Drawing for the job (mm, zero at the part's lowest x, y, z). A direction names the side the tool comes from. Round coordinates to 2 decimals unless told otherwise and drop trailing zeros. Loops run counter-clockwise (first coordinate to the right, second up) from the corner with the lowest first, then second, coordinate; pieces in that order, holes last. Notation, with made-up numbers: (61.5, 32) - (75.5, 32) arc R21 cw to (75.5, 61) - close; hole circle Ø6 at (61.5, 72). An arc over 180 degrees is marked (long way). Put each result on its own line as item: value.
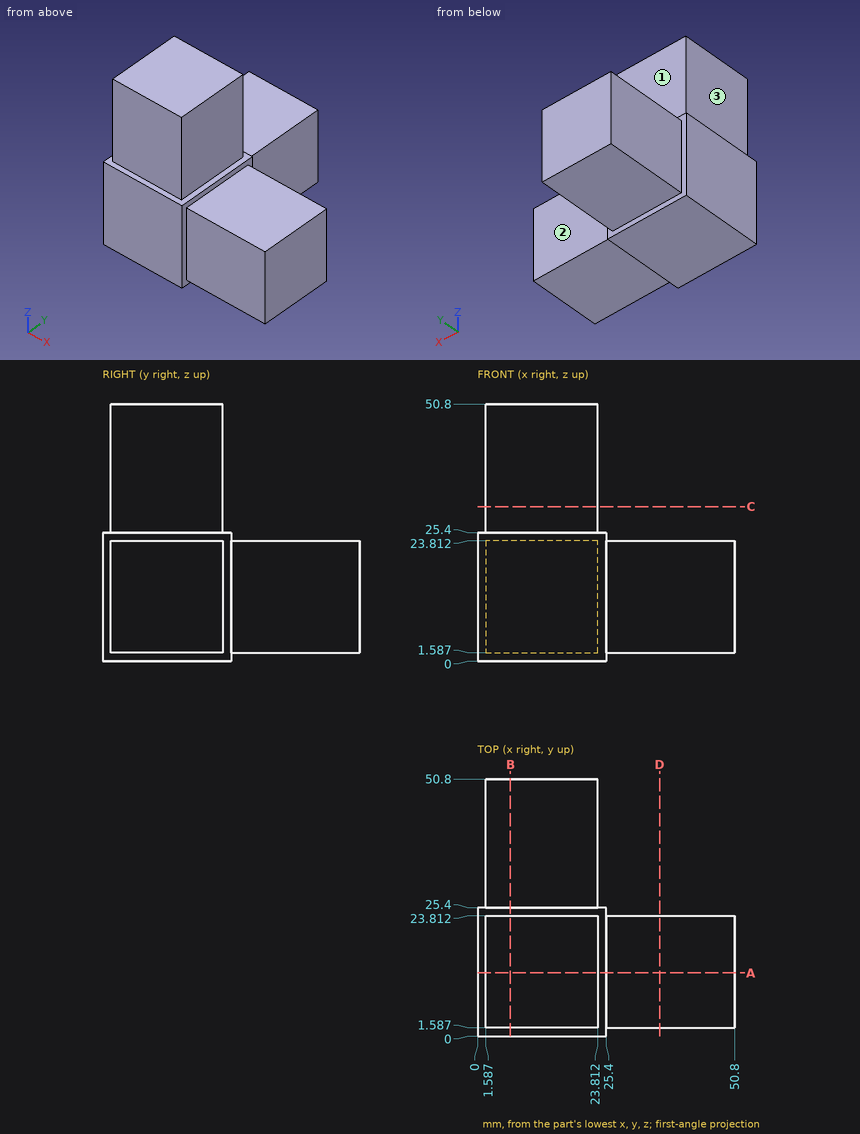
1. Probe line 1 along Y through (x, z) = (23, 32.5). List the from-to ranges inside material, lowest first. Write a range as [from, to].
A:
line 1: y = [1.59, 23.81]
2. Band-saw the part on A-A (y = 12.5). List the corners of the cut face in (x, z).
A:
outline: (0, 0) - (25.4, 0) - (25.4, 1.59) - (50.8, 1.59) - (50.8, 23.81) - (25.4, 23.81) - (25.4, 25.4) - (23.81, 25.4) - (23.81, 50.8) - (1.59, 50.8) - (1.59, 25.4) - (0, 25.4) - close
3. Tool access for the marked faces 1, 2 and 3: list every direction of +Z, -Z, +X, -X, +Y, -Y with a clear straight run to the whole face (end or side of a thin tool).
A:
face 1: +Z, +X, -X, +Y
face 2: +Z, -Z, +X, +Y
face 3: +Z, -X, +Y, -Y
4. Pin check, flat tips, straight feed: P1, Ø18, axis at y = 12, z = 40.5, coming from the +X side; P2, Ø6.5, axis at x = 18, z = 32, coming from the +Y side; P3, Ø18, axis at x = 37, y = 17.5, coming from the -Z side. Stop position of each tip, or through.
A:
P1: stops at x = 23.81
P2: stops at y = 23.81
P3: stops at z = 1.59
5. Band-saw the part on C-C (z = 30.5). List the corners of the cut face in (x, y).
A:
outline: (1.59, 1.59) - (23.81, 1.59) - (23.81, 23.81) - (1.59, 23.81) - close
